```python
from build123d import *

# Parameters (mm, degrees)
SKETCH5_W                    = 235.204
SKETCH5_H                    = 50.8
BOSS_EXTRUDE3_DEPTH          = 7.62
CUT_EXTRUDE3_DEPTH           = 6.35
F_10_0_1935_DIAMETER_HOLE1_D = 4.9149


with BuildPart() as part:
    # Sketch5 → Boss-Extrude3 (new body)
    with BuildSketch(Plane.XY):
        with Locations((-117.602, 25.4)):
            Rectangle(SKETCH5_W, SKETCH5_H)
    extrude(amount=BOSS_EXTRUDE3_DEPTH)

    # Sketch6 → Cut-Extrude3 (cut)
    with BuildSketch(Plane.XY.offset(7.62)):
        with BuildLine():
            Line((-48.26, 11.176), (-175.975043584, 11.176))
            ThreePointArc((-175.975043584, 11.176), (-190.199043584, 25.4), (-175.975043584, 39.624))
            Line((-175.975043584, 39.624), (-48.26, 39.624))
            ThreePointArc((-48.26, 39.624), (-34.036, 25.4), (-48.26, 11.176))
        make_face()
    extrude(amount=-CUT_EXTRUDE3_DEPTH, mode=Mode.SUBTRACT)

    # #10 (0.1935) Diameter Hole1 (through all)
    with Locations(Plane(origin=(-198.501, 45.72, 7.62), x_dir=(1, 0, 0), z_dir=(0, 0, 1))):
        with Locations((0, 0), (40.386, 0), (80.772, 0), (121.158, 0), (161.544, 0), (-20.193, -41.171520692), (20.2438, -41.171520692), (60.6806, -41.171520692), (101.1174, -41.171520692), (141.5542, -41.171520692), (181.991, -41.171520692)):
            Hole(F_10_0_1935_DIAMETER_HOLE1_D / 2)


solid = part.part
```
Geometry check sheet. Reference: the model listing, model coordinates, mm. A direction names the side the tool comes from. Coordinates: 2 decimals unless noted, no trailing zeros. Order: outer loops, then holes, each group sorted by start corner. A loop starts at its lowest first (then second) coordinate and runs counter-clockwise, first axis right, second up. Notation, with made-up numbers: (71, 25.25) - (130, 25.25) arc R27 cw to (130, 61.25) - close; hole circle Ø3 at (-33.75, -7.75). An arc over 180 degrees is marked (long way). Answer as a JSON object with one key per item and string values. Group by question number.
Item 1: Tool access check on faces 1 (the face through (-190.196, 25.087, 4.489)), 2 (the face through (-140.164, 5.287, 3.757)). Record the directions out of +Z, -Z, +X, -X, +Y, -Y that give a thin tool (end or side, any length) a straight path to the whole face; none if there is none.
Item 2: Sectioned sample at B-B, the plane x = -16.51. Record the cut outline in (y, z).
Item 3: Draft check along Y on faces 3 (the face through (-119, 50.8, 4)), 4 (the face through (-119, 0, 4)), 5 (the face through (-235.204, 25, 4)), 6 (the face through (-111, 11.176, 4)). Enter one of: +Y half, -Y half, draft (parallel to the pull), parting line (faces both ways), or undercut.
Item 4: Scan lines: probe 1 along X at (y, z) = (46, 4.5); probe 2 along Y at (x, z) = (-122.5, 6.25); probe 3 along Y at (x, z) = (-16.51, 2.5). Record each from-to range of solid material in increasing order.
Item 5: Sectioned sample at D-D, the plane y = 25.4. Record the cut outline in (x, z), and give its area (3 significant figures).
Item 6: Sectioned sample at C-C, the plane x = -111. Record the cut outline in (y, z).
Item 7: Sectioned sample at A-A, the plane y = 45.72. Record the cut outline in (x, z).
Resolved:
{
 "1": {"face 1": "+Z", "face 2": "+Z, -Z"},
 "2": {"outline": "(0, 0) - (2.09, 0) - (2.09, 7.62) - (0, 7.62) - close; (7.01, 0) - (50.8, 0) - (50.8, 7.62) - (7.01, 7.62) - close"},
 "3": {"face 3": "+Y half", "face 4": "-Y half", "face 5": "draft", "face 6": "undercut"},
 "4": {"probe 1": "-235.2 to -200.94, -196.06 to -160.56, -155.67 to -120.17, -115.29 to -79.78, -74.9 to -39.4, -34.52 to 0", "probe 2": "0 to 11.18, 39.62 to 50.8", "probe 3": "0 to 2.09, 7.01 to 50.8"},
 "5": {"outline": "(-235.2, 0) - (0, 0) - (0, 7.62) - (-34.04, 7.62) - (-34.04, 1.27) - (-190.2, 1.27) - (-190.2, 7.62) - (-235.2, 7.62) - close", "area": "801 mm^2"},
 "6": {"outline": "(0, 0) - (50.8, 0) - (50.8, 7.62) - (39.62, 7.62) - (39.62, 1.27) - (11.18, 1.27) - (11.18, 7.62) - (0, 7.62) - close"},
 "7": {"outline": "(-235.2, 0) - (-200.96, 0) - (-200.96, 7.62) - (-235.2, 7.62) - close; (-196.04, 0) - (-160.57, 0) - (-160.57, 7.62) - (-196.04, 7.62) - close; (-155.66, 0) - (-120.19, 0) - (-120.19, 7.62) - (-155.66, 7.62) - close; (-115.27, 0) - (-79.8, 0) - (-79.8, 7.62) - (-115.27, 7.62) - close; (-74.89, 0) - (-39.41, 0) - (-39.41, 7.62) - (-74.89, 7.62) - close; (-34.5, 0) - (0, 0) - (0, 7.62) - (-34.5, 7.62) - close"}
}
